Geometry check sheet. Reference: the model listing, model coordinates, mm. Face numbers are marked on the shaded views. A direction names the side the tool comes from. Give positions to 0.01 mm unless a question says otherwise; leave off trailing zeros. Loops run counter-clockwise (first coordinate to the right, second up) from the corner with the lowest first, then second, coordinate; pieces in that order, holes last. Notation, with made-up numbers: (73, 35.25) -> (127, 35.25) arc R19 cw to (127, 40.25) -> close; hole circle Ø1 at (67.25, -21.5). An arc over 180 degrees is marked (long way). One line per item, written item: value. Start each with the question number.
(1) Gauge pin test, flat ends, axial feed: pin 1 Ø3 at (y, z) = (17.5, 3) entering from -X (3 decimals); pin 2 Ø1.5 at (y, z) = (69, 6.5) entering from -X; pin 3 Ø13.5 at (x, y) = (205, 46) entering from +Z. Record the tip position at first contact, or that the pin passes through.
(2) Sectioned sample at B-B, the plane x = 200. Record the cut outline in (y, z).
(3) Draft check along X on the marked faces 1, 2 and 3. Enter one of: pulls with the +X half, pulls with the -X half, needs draft (parallel to the pull), parting line crosses it, or undercut.
(4) Scan lines: line 1 along X through (y, z) = (35, 17.5); line 2 along X through (y, z) = (30, 19); line 3 along Z through (x, y) = (47, 55.5). Record each from-to range of solid material in increasing order. Write a range as from..to.
(5) Tool access check on the marked faces 4 and 5. Record the directions out of +Z, -Z, +X, -X, +Y, -Y that give a thin tool (end or side, any length) a straight path to the whole face; none if there is none.
(6) Sectioned sample at A-A, the plane z = 7.25. Record the cut outline in (x, y), then the cut area to 3 significant figures.
from build123d import *

# Parameters (mm, degrees)
F0_W     = 240
F0_H     = 80
F1_DEPTH = 20
F2_R     = 25
F3_DEPTH = 16
F3_TAPER = 10
F4_R     = 20


with BuildPart() as f1:
    # F0 (on Top) → F1 (new body)
    with BuildSketch(Plane.XY):
        with Locations((120, 40)):
            Rectangle(F0_W, F0_H)
    extrude(amount=F1_DEPTH)

    # F2 (on face) → F3 (cut)
    with BuildSketch(Plane.XY.offset(20)):
        with Locations((40, 40)):
            Circle(F2_R)
        with Locations((120, 40)):
            Circle(F2_R)
        with Locations((200, 40)):
            Circle(F2_R)
    extrude(amount=-F3_DEPTH, taper=F3_TAPER, mode=Mode.SUBTRACT)

    # F4
    f4_edges = [f1.edges().sort_by_distance(p)[0] for p in [
        (240, 0, 10),
        (240, 80, 10),
        (0, 80, 10),
        (0, 0, 10),
    ]]
    fillet(f4_edges, radius=F4_R)


solid = f1.part
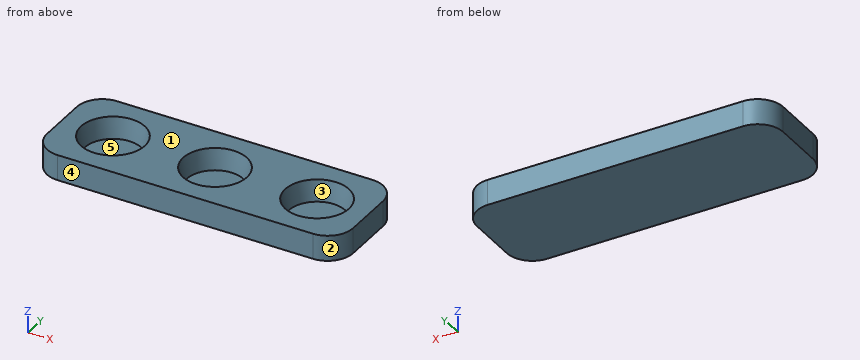
Calculated:
1. pin 1: stops at x = 0.025
1. pin 2: stops at x = 1.78
1. pin 3: stops at z = 4
2. outline: (0, 0) -> (80, 0) -> (80, 20) -> (65, 20) -> (62.18, 4) -> (17.82, 4) -> (15, 20) -> (0, 20) -> close
3. face 1: needs draft
3. face 2: pulls with the +X half
3. face 3: undercut
4. line 1: x = 0..15.96, 64.04..95.96, 144.04..175.96, 224.04..240
4. line 2: x = 0..17.28, 62.72..97.28, 142.72..177.28, 222.72..240
4. line 3: z = 0..4
5. face 4: +Z, -Z, +X, -X, -Y
5. face 5: +Z
6. outline: (0, 20) arc R20 ccw to (20, 0) -> (220, 0) arc R20 ccw to (240, 20) -> (240, 60) arc R20 ccw to (220, 80) -> (20, 80) arc R20 ccw to (0, 60) -> close; hole circle Ø45.5 at (40, 40); hole circle Ø45.5 at (120, 40); hole circle Ø45.5 at (200, 40)
6. area: 14,000 mm2
